Build history of the part. All positions in model axes, mm. Round coordinates to 2 decimals unless told otherwise and drop trailing zeros. Order: outer loops, then holes, each group sorted by start corner. A loop starts at its lowest first (then second) coordinate and runs counter-clockwise, first axis right, second up. Notation, with made-up numbers: (-16, -3) -> (0, -3) arc R29 cw to (0, 21) -> close; hole circle Ø5 at (58.25, 56). An arc over 180 degrees is marked (long way). Answer as CSV lines item,"result". Start each with the question number.
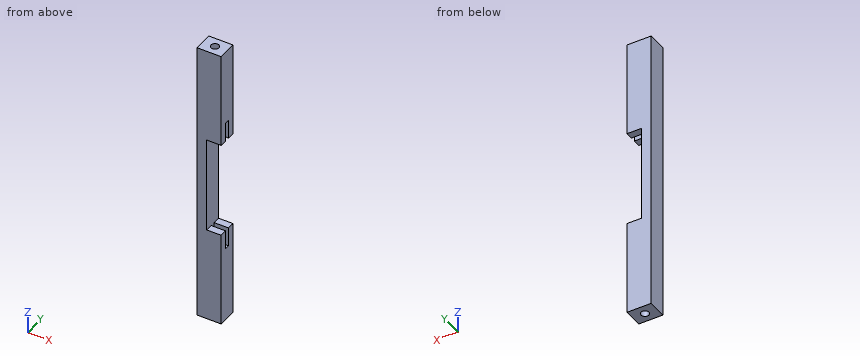
Autodesk Inventor part; units mm, degrees
ref_plane "YZ Plane" through (0, 0, 0) normal (1, 0, 0) x (0, 1, 0)
ref_plane "XZ Plane" through (0, 0, 0) normal (0, 1, 0) x (-1, 0, 0)
ref_plane "XY Plane" through (0, 0, 0) normal (0, 0, 1) x (1, 0, 0)
sketch "Sketch3" plane through (0, 0, 0) normal (1, 0, 0) x (0, 1, 0)
  line L0 (-4, 59.5) -> (4, 59.5)
  line L1 (4, 59.5) -> (4, -59.5)
  line L2 (4, -59.5) -> (-4, -59.5)
  line L3 (-4, -59.5) -> (-4, 59.5)
  line L4 (-67.3512, -62.0209) -> (6.0524, -62.0209)
  line L5 (-86.0704, 69.3717) -> (-9.6617, 69.3717)
  line L6 (-9.4707, -54.67) -> (-85.8794, -54.67)
  point P0 (0, 0)
  dimension "d7" = 119
  dimension "d8" = 59.5
  dimension "d9" = 8
  dimension "d10" = 4
  dimension "d50" = 124.0417
extrude "Extrusion1" add sketch "Sketch3" along normal blind 4
sketch "Sketch4" plane through (4, 0, 0) normal (1, 0, 0) x (0, 0, -1)
  line L0 (-59.5, 4) -> (59.5, 4)
  line L1 (-59.5, -4) -> (-59.5, 4)
  line L2 (59.5, -4) -> (-59.5, -4)
  line L3 (59.5, 4) -> (59.5, -4)
  line L4 (-59.5, 4) -> (-20, 4)
  line L5 (-20, -4) -> (-59.5, -4)
  line L6 (-59.5, -4) -> (-59.5, 4)
  line L7 (59.5, 4) -> (59.5, -4)
  line L8 (-20, 4) -> (-20, 1)
  line L9 (-20, 1) -> (-28, 1)
  line L10 (-28, 1) -> (-28, -1)
  line L11 (-28, -1) -> (-20, -1)
  line L12 (-20, -1) -> (-20, -4)
  line L13 (0, -4) -> (0, 4)
  line L14 (59.5, 4) -> (20, 4)
  line L15 (20, 1) -> (28, 1)
  line L16 (28, 1) -> (28, -1)
  line L17 (28, -1) -> (20, -1)
  line L18 (20, -1) -> (20, -4)
  line L19 (20, 4) -> (20, 1)
  line L20 (20, -4) -> (59.5, -4)
  point P0 (0, 0)
  dimension "d20" = 28
  dimension "d21" = 2
  dimension "d22" = 1
  dimension "d23" = 20
  dimension "d24" = 20
  dimension "d25" = 20
  dimension "d26" = 20
  dimension "d27" = 1
  dimension "d28" = 1
  dimension "d29" = 28
extrude "Extrusion3" add sketch "Sketch4" along normal blind 6 contours L0 L8 L9 L10 L11 L12 L2 L1 | L0 L3 L2 L18 L17 L16 L15 L19
sketch "Sketch6" plane through (0, -4, 59.5) normal (0, 0, 1) x (1, 0, 0)
  line L0 (0, 8) -> (10, 8)
  line L1 (0, 0) -> (0, 8)
  point P0 (0, 4)
  point P1 (5, 4)
  dimension "d32" = 4
  dimension "d33" = 5
hole "Hole1" at (5, 0, 59.5) direction (0, 0, -1) diameter 3.242 depth 8.5 tip angle 118
sketch "Sketch7" plane through (0, -4, -59.5) normal (0, 0, -1) x (-1, 0, 0)
  line L0 (0, 0) -> (-10, 0)
  line L1 (0, 8) -> (0, 0)
  point P0 (0, 4)
  point P1 (-5, 4)
  dimension "d41" = 5
  dimension "d42" = 4
hole "Hole2" at (5, 0, -59.5) direction (0, 0, 1) diameter 3.242 depth 8.5 tip angle 118
properties part number "feet"
Q1. Flat gauge pins, fed straight in: pin 1 Ø1.5 at (y, z) = (1.5, -1.5) entering from +X; pin 2 Ø1.6 at (x, y) = (6.5, 0.5) entering from -Z; pin 3 Ø3 at (x, y) = (5, 0) entering from -Z. Where does each tip first touch, or does it go through?
Q2. Slice it at C-C, the plane z = -6.5. Write the cut outline in (x, y).
Q3. Slice it at B-B, the plane z = 26.5. Write the cut outline in (x, y).
Q4. Slice it at A-A, the plane y = 2.75. Write the cut outline in (x, z).
Q5. Probe L1, parallel to X at y = 0, z = 55.25; L2, parallel to Z at x = 8.25, y = 0.75; L3, parallel to Y at x = 5, z = 56.25. List the from-to ranges inside material, lowest first.
Solutions:
1,pin 1,"stops at x = 4"
1,pin 2,"stops at z = -59.5"
1,pin 3,"stops at z = -50.93"
2,outline,"(0, -4) -> (4, -4) -> (4, 4) -> (0, 4) -> close"
3,outline,"(0, -4) -> (10, -4) -> (10, -1) -> (4, -1) -> (4, 1) -> (10, 1) -> (10, 4) -> (0, 4) -> close"
4,outline,"(0, -59.5) -> (10, -59.5) -> (10, -20) -> (4, -20) -> (4, 20) -> (10, 20) -> (10, 59.5) -> (0, 59.5) -> close"
5,L1,"x = 0 to 3.38, 6.62 to 10"
5,L2,"z = -59.5 to -28, 28 to 59.5"
5,L3,"y = -4 to -1.62, 1.62 to 4"
